Print and shaded views of the part. All mm, measured from the part's lowest x, y and z. A direction names the side the tool comes from. Round coordinates to 2 decimals unless told otherwise and drop trailing zeros. Order: outer loops, then holes, each group sorted by start corner. A loop starts at its lowest first (then second) coordinate and runs counter-clockwise, first axis right, second up.
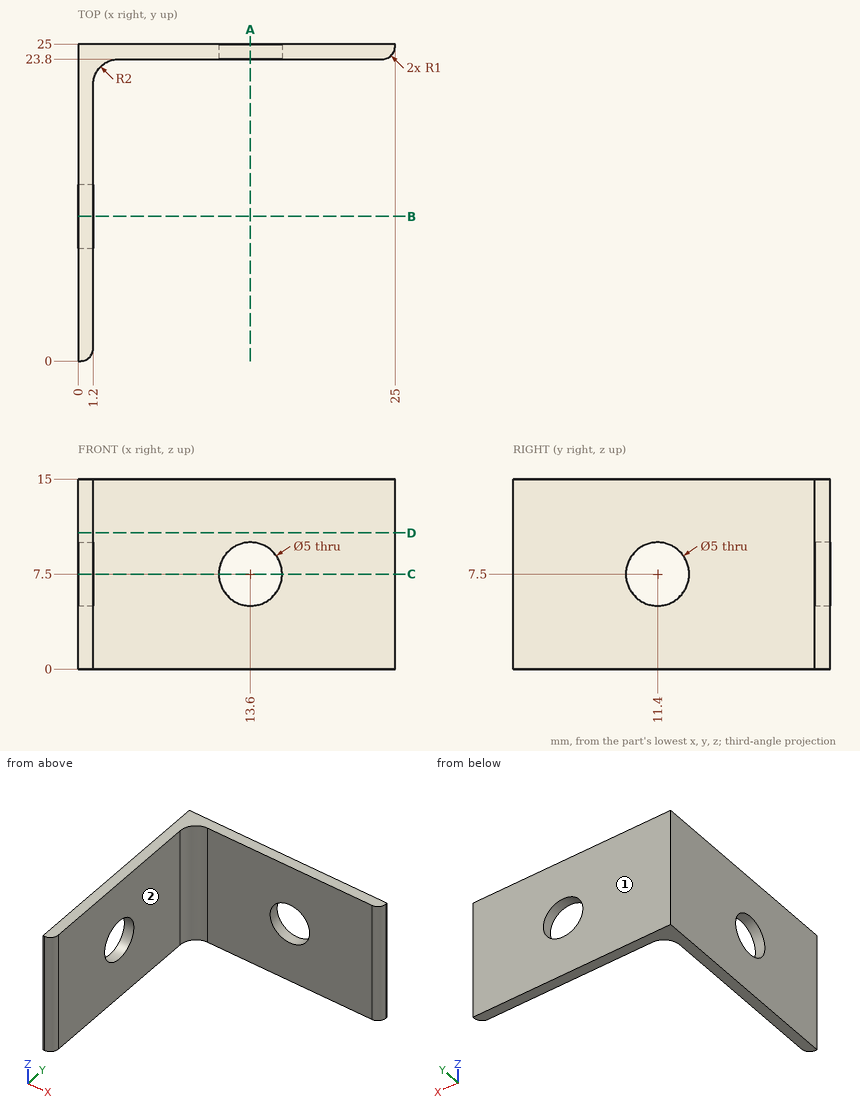
1. Cut at B-B, the plane y = 11.4. Write the cut outline in (x, z).
2. Cut at A-A, the plane x = 13.6. Write the cut outline in (y, z), and give its area (3 significant figures).
3. Drill centre lines: line 1 (X direction, y = 7.5, z = 2.25); line 2 (Y direction, x = 9.5, z = 4); line 3 (Z direction, x = 0.7, y = 11.4). Where is each one in solid material? Low to high.
4. Pin check, flat tips, straight feed: P1, Ø4.5, axis at y = 11, z = 8.5, coming from the +X side; P2, Ø6, axis at x = 13.6, z = 7.5, coming from the -Y side. Stop position of each tip, or through.
5. Cut at C-C, the plane z = 7.5. Write the cut outline in (x, y), and give its area (3 significant figures).
6. Cut at D-D, the plane z = 10.75. Write the cut outline in (x, y), and give its area (3 significant figures).
7. Tool access for the marked faces 1 and 2: list every direction of +Z, -Z, +X, -X, +Y, -Y with a clear straight run to the whole face (end or side of a thin tool).
Outcome:
1. outline: (0, 0) - (1.2, 0) - (1.2, 5) - (0, 5) - close; (0, 10) - (1.2, 10) - (1.2, 15) - (0, 15) - close
2. outline: (23.8, 0) - (25, 0) - (25, 5) - (23.8, 5) - close; (23.8, 10) - (25, 10) - (25, 15) - (23.8, 15) - close
2. area: 12.0 mm2
3. line 1: x = 0 to 1.2
3. line 2: y = 23.8 to 25
3. line 3: z = 0 to 5, 10 to 15
4. P1: stops at x = 1.2
4. P2: stops at y = 23.8
5. outline: (0, 0) - (0.2, 0) arc R1 ccw to (1.2, 1) - (1.2, 8.9) - (0, 8.9) - close; (0, 13.9) - (1.2, 13.9) - (1.2, 21.8) arc R2 cw to (3.2, 23.8) - (11.1, 23.8) - (11.1, 25) - (0, 25) - close; (16.1, 23.8) - (24, 23.8) arc R1 ccw to (25, 24.8) - (25, 25) - (16.1, 25) - close
5. area: 47.0 mm2
6. outline: (0, 0) - (0.2, 0) arc R1 ccw to (1.2, 1) - (1.2, 21.8) arc R2 cw to (3.2, 23.8) - (24, 23.8) arc R1 ccw to (25, 24.8) - (25, 25) - (0, 25) - close
6. area: 59.0 mm2
7. face 1: +Z, -Z, +X, -X, +Y
7. face 2: +Z, -Z, +X, -Y
